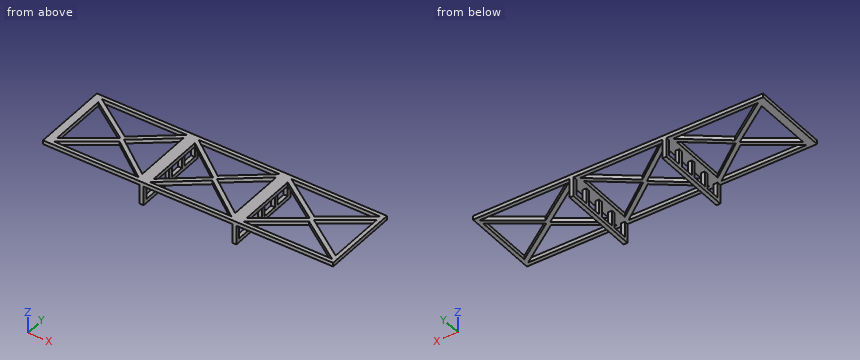
from build123d import *

# Parameters (mm, degrees)
F1_DEPTH      = 20
F3_DEPTH      = 2
F4_W          = 7.5
F4_H          = 8
F5_DEPTH      = 2
F5_DEPTH_BACK = 48


with BuildPart() as f1:
    # F0 (on Front) → F1 (new body, symmetric)
    with BuildSketch(Plane.XZ):
        Polygon((75, 0), (-75, 0), (-75, -2), (-25, -2), (-25, -12), (-23, -12), (-23, -2), (23, -2), (23, -12), (25, -12), (25, -2), (75, -2), align=None)
    extrude(amount=F1_DEPTH, both=True)

    # F2 (on face) → F3 (cut, through all)
    with BuildSketch(Plane(origin=(0, 0, -2), x_dir=(1, 0, 0), z_dir=(0, 0, -1))):
        Polygon((-27, 18), (-71, 18), (-48, 2), align=None)
        Polygon((21, 18), (-21, 18), (0, 2), align=None)
        Polygon((73, 18), (27, 18), (50, 2), align=None)
        Polygon((-27, -18), (-48, -2), (-71, -18), align=None)
        Polygon((21, -18), (0, -2), (-21, -18), align=None)
        Polygon((73, -18), (50, -2), (27, -18), align=None)
        Polygon((-49, 0), (-71, 15.3043478261), (-71, -15.3043478261), align=None)
        Polygon((-27, -15.2380952381), (-27, 15.2380952381), (-47, 0), align=None)
        Polygon((-1, 0), (-21, 15.2380952381), (-21, -15.2380952381), align=None)
        Polygon((21, -15.2380952381), (21, 15.2380952381), (1, 0), align=None)
        Polygon((48.9047619048, 0), (27, 15.2380952381), (27, -15.2380952381), align=None)
        Polygon((73, -15.2380952381), (73, 15.2380952381), (51.0952380952, 0), align=None)
    extrude(amount=-F3_DEPTH, mode=Mode.SUBTRACT)

    # F4 (on face) → F5 (cut, two sides)
    with BuildSketch(Plane(origin=(23, 0, 0), x_dir=(0, -1, 0), z_dir=(-1, 0, 0))) as f5_sk:
        with Locations((14.25, -6)):
            Rectangle(F4_W, F4_H)
        with Locations((4.75, -6)):
            Rectangle(F4_W, F4_H)
        with Locations((-4.75, -6)):
            Rectangle(F4_W, F4_H)
        with Locations((-14.25, -6)):
            Rectangle(F4_W, F4_H)
    extrude(amount=-F5_DEPTH, mode=Mode.SUBTRACT)
    extrude(f5_sk.sketch, amount=F5_DEPTH_BACK, mode=Mode.SUBTRACT)


solid = f1.part
Source: CAD feature listing. Evaluate the final solid. Frame: model axes, mm. Round coordinates to 2 decimals unless told otherwise and drop trailing zeros. Loops run counter-clockwise (first coordinate to the right, second up) from the corner with the lowest first, then second, coordinate; pieces in that order, holes last. Notation, with made-up numbers: (-15.75, 72.5) - (-11.75, 72.5) arc R38 cw to (-11.75, 111.5) - close; hole circle Ø10 at (58.25, 44.25). An arc over 180 degrees is marked (long way). Write item = value, one per line. Start each with the question number.
(1) Section query B-B, the plane z = -4.75. State how many separate pieces and enclosed holes the cut face has, plus the area to 3 significant figures.
(2) Pin query (flat end, axial travel): pin 1 (5 mm diameter, centred on x = 38.5, y = 12, fed in from +Z); pin 2 (10 mm diameter, centred on x = -54.5, y = -15, fed in from -Z). Return the tip coordinate at first contact, or that it passes through.
(3) Section query D-D, the plane x = -62. Output: boundary loops of the cut face in (y, z), plus the area to 3 significant figures.
(4) Section query A-A, the plane x = 31. Output: boundary loops of the cut face in (y, z), plus the area to 3 significant figures.
(5) Ray query, line 1 along X through (y, z) = (0.5, -5); line 2 along Y through (x, z) = (53.5, -0.5); line 3 along Y through (x, z) = (28.5, -0.75). Return the intervals inside material, ascending. Write a range as from..to.
Conclusion:
q1.separate_pieces = 10
q1.enclosed_holes = 0
q1.area = 40.0 mm2
q2.pin_1 = 0
q2.pin_2 = -2
q3.outline = (-20, -2) - (-18, -2) - (-18, 0) - (-20, 0) - close; (-11.74, -2) - (-9.04, -2) - (-9.04, 0) - (-11.74, 0) - close; (9.04, -2) - (11.74, -2) - (11.74, 0) - (9.04, 0) - close; (18, -2) - (20, -2) - (20, 0) - (18, 0) - close
q3.area = 18.8 mm2
q4.outline = (-20, -2) - (-18, -2) - (-18, 0) - (-20, 0) - close; (-15.22, -2) - (-12.46, -2) - (-12.46, 0) - (-15.22, 0) - close; (12.46, -2) - (15.22, -2) - (15.22, 0) - (12.46, 0) - close; (18, -2) - (20, -2) - (20, 0) - (18, 0) - close
q4.area = 19.0 mm2
q5.line_1 = -25..-23, 23..25
q5.line_2 = -20..-18, -4.43..-1.67, 1.67..4.43, 18..20
q5.line_3 = -20..-18, -16.96..-14.19, 14.19..16.96, 18..20
